Part model, mm, in its own coordinate system. Face numbers are marked on the shaded views. A direction names the side the tool comes from. Round coordinates to 2 decimals unless told otherwise and drop trailing zeros. Loops run counter-clockwise (first coordinate to the right, second up) from the corner with the lowest first, then second, coordinate; pieces in that order, holes last.
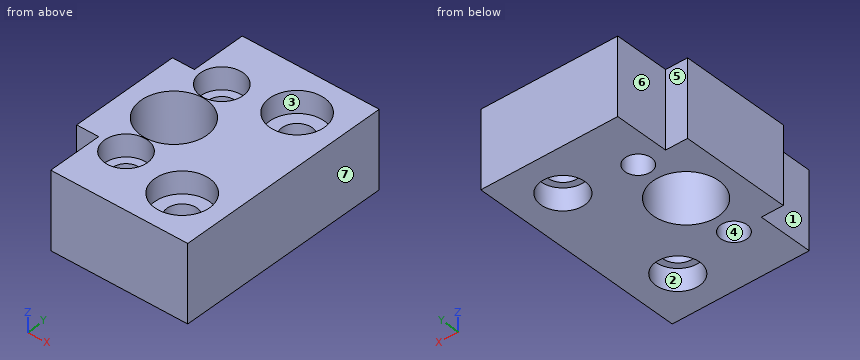
Autodesk Inventor part; units mm, degrees
ref_plane "YZ Plane" through (0, 0, 0) normal (1, 0, 0) x (0, 1, 0)
ref_plane "XZ Plane" through (0, 0, 0) normal (0, 1, 0) x (-1, 0, 0)
ref_plane "XY Plane" through (0, 0, 0) normal (0, 0, 1) x (1, 0, 0)
sketch "Sketch1" plane through (0, 0, 0) normal (0, 0, 1) x (1, 0, 0)
  line L0 (10, -10) -> (-10, -10)
  line L1 (-10, -10) -> (-10, 10)
  line L2 (-10, 10) -> (10, 10)
  line L3 (10, 10) -> (10, -10)
  circle A0 centre (0, 5) radius 1.2
  circle A1 centre (0, -5) radius 1.2
  circle A2 centre (0, 0) radius 3
  dimension "d0" = 10
  dimension "d1" = 10
  dimension "d2" = 10
  dimension "d3" = 10
  dimension "d4" = 5
  dimension "d5" = 5
  dimension "d6" = 2.4
  dimension "d7" = 2.4
  dimension "d8" = 6
extrude "Extrusion1" add sketch "Sketch1" along normal blind 5
sketch "Sketch2" plane through (0, 0, 5) normal (0, 0, 1) x (1, 0, 0)
  line L0 (0, 0) -> (-1.3346, -1.3533)
  circle A0 centre (6, -6) radius 2.5
  circle A1 centre (6, 6) radius 2.5
  line L1 (10, -10) -> (10, 10)
  line L2 (-10, -10) -> (10, -10)
  line L3 (10, 10) -> (-10, 10)
  dimension "d34" = 4
  dimension "d35" = 4
  dimension "d36" = 4
  dimension "d37" = 4
  dimension "d38" = 5
  dimension "d39" = 5
extrude "Extrusion2" cut sketch "Sketch2" against normal blind 1
sketch "Sketch7" plane through (0, 0, 0) normal (0, 0, -1) x (-1, 0, 0)
  circle A0 centre (-6, 6) radius 2.5
  circle A1 centre (-6, 6) radius 1.375
  circle A2 centre (-6, -6) radius 2.5
  circle A3 centre (-6, -6) radius 1.375
  point P0 (0, 0)
  dimension "d40" = 2.75
  dimension "d41" = 2.75
extrude "Extrusion6" cut sketch "Sketch7" against normal blind 5 contours A1 | A3
sketch "Sketch8" plane through (0, 0, 5) normal (0, 0, 1) x (1, 0, 0)
  line L0 (10, 10) -> (-10, 10)
  line L1 (10, 10) -> (2.5, 10)
  line L2 (2.5, 10) -> (2.5, 2.5)
  line L3 (2.5, 2.5) -> (10, 2.5)
  line L4 (10, 2.5) -> (10, 10)
  line L5 (10, -10) -> (10, 10)
  line L6 (10, -10) -> (2.5, -10)
  line L7 (2.5, -10) -> (2.5, -2.5)
  line L8 (2.5, -2.5) -> (10, -2.5)
  line L9 (10, -2.5) -> (10, -10)
  line L10 (10, -2.5) -> (5, -2.5)
  line L11 (5, -2.5) -> (5, 2.5)
  line L12 (5, 2.5) -> (10, 2.5)
  line L13 (10, 2.5) -> (10, -2.5)
  circle A0 centre (6, 6) radius 2.5
  circle A1 centre (6, 6) radius 2.5
  circle A2 centre (6, -6) radius 2.5
  circle A3 centre (6, -6) radius 2.5
  point P0 (0, 0)
  point P1 (2.5, 10)
  dimension "d44" = 7.5
  dimension "d45" = 7.5
  dimension "d46" = 7.5
  dimension "d47" = 7.5
  dimension "d48" = 5
extrude "Extrusion7" add sketch "Sketch8" along normal blind 2
sketch "Sketch9" plane through (0, 0, 0) normal (0, 0, -1) x (-1, 0, 0)
  circle A0 centre (-6, 6) radius 1.375
  circle A1 centre (-6, 6) radius 2
  circle A2 centre (-6, -6) radius 1.375
  circle A3 centre (-6, -6) radius 2
  point P0 (0, 0)
  dimension "d51" = 4
  dimension "d52" = 4
extrude "Extrusion8" cut sketch "Sketch9" against normal blind 2 contours A0 | A1 | A2 | A3
sketch "Sketch10" plane through (0, 0, 0) normal (0, 0, -1) x (-1, 0, 0)
  line L0 (-2.5, 10) -> (10, 10)
  line L1 (10, -10) -> (-2.5, -10)
  line L2 (10, 10) -> (5, 10)
  line L3 (5, 10) -> (5, -10)
  line L4 (5, -10) -> (10, -10)
  line L5 (10, -10) -> (10, 10)
  line L6 (5, 10) -> (2.5, 10)
  line L7 (2.5, 10) -> (2.5, 5)
  line L8 (2.5, 5) -> (5, 5)
  line L9 (5, 5) -> (5, 10)
  line L10 (5, -10) -> (2.5, -10)
  line L11 (2.5, -10) -> (2.5, -5)
  line L12 (2.5, -5) -> (5, -5)
  line L13 (5, -5) -> (5, -10)
  point P0 (0, 0)
  point P1 (2.5, 10)
  dimension "d55" = 5
  dimension "d56" = 2.5
  dimension "d57" = 5
  dimension "d58" = 5
  dimension "d59" = 2.5
extrude "Extrusion9" cut sketch "Sketch10" against normal blind 10
sketch "Sketch12" plane through (6, -6, 4) normal (0, 0, 1) x (1, 0, 0)
  circle A0 centre (0, 0) radius 1.375
  circle A1 centre (0, 0) radius 2.5
  circle A2 centre (0, 12) radius 2
  circle A3 centre (0, 12) radius 1.375
  circle A4 centre (0, 12) radius 2.5
  point P0 (-6, 6)
extrude "Extrusion11" add sketch "Sketch12" along normal blind 1 contours A1 | A2 | A4
sketch "Sketch13" plane through (0, 0, 5) normal (0, 0, 1) x (1, 0, 0)
  point P0 (0, 0)
sketch "Sketch14" plane through (0, 0, 5) normal (0, 0, 1) x (1, 0, 0)
  line L0 (-2.5, -5) -> (-2.5, -10)
  line L1 (-2.5, -10) -> (2.5, -10)
  line L2 (2.5, -10) -> (2.5, -2.5)
  line L3 (2.5, -2.5) -> (5, -2.5)
  line L4 (5, -2.5) -> (5, 2.5)
  line L5 (5, 2.5) -> (2.5, 2.5)
  line L6 (2.5, 2.5) -> (2.5, 10)
  line L7 (2.5, 10) -> (-2.5, 10)
  line L8 (-2.5, 10) -> (-2.5, 5)
  line L9 (-2.5, 5) -> (-5, 5)
  line L10 (-5, 5) -> (-5, -5)
  line L11 (-5, -5) -> (-2.5, -5)
  circle A0 centre (0, 0) radius 3
  circle A1 centre (0, -5) radius 1.2
  circle A2 centre (0, 5) radius 1.2
  circle A3 centre (0, -5) radius 1.95
  circle A4 centre (0, 5) radius 1.95
  dimension "d80" = 3.9
  dimension "d81" = 3.9
extrude "Extrusion12" add sketch "Sketch14" along normal blind 2 contours L11 L10 L9 L8 L7 L6 L5 L4 L3 L2 L1 L0
sketch "Sketch15" plane through (-5, -5, 0) normal (-1, 0, 0) x (0, 0, 1)
  line L0 (0, 10) -> (7, 10)
  line L1 (0, 0) -> (0, 10)
  line L2 (0, 0) -> (7, 0)
  line L3 (7, 10) -> (7, 0)
  point P0 (0, 5)
extrude "Extrusion13" cut sketch "Sketch15" against normal blind 0.5
equation "\"d7\" = d6"
equation "\"d39\" = d38"
equation "\"d45\" = d44"
equation "\"d46\" = d45"
equation "\"d52\" = d51"
equation "\"d81\" = d80"
properties part number "MotorMount"
1) Slice it at D-D, the plane y = -2. Give the cut face in (x, z).
Values:
outline: (-4.5, 0) - (-2.24, 0) - (-2.24, 7) - (-4.5, 7) - close; (2.24, 0) - (10, 0) - (10, 7) - (2.24, 7) - close
2) Drop flat-ended pins along their axis: pin 1 Ø3.5 at (x, y) = (6, 6) entering from -Z; pin 2 Ø3 at (x, y) = (0, -5) entering from +Z; pin 3 Ø5 at (x, y) = (0, 0) entering from -Z; pin 4 Ø1.5 at (y, z) = (6.5, 2.5) entering from -X. Give the stop position or say it passes through.
Values:
pin 1: stops at z = 2
pin 2: stops at z = 5
pin 3: passes through
pin 4: stops at x = -2.5
3) Tool access for the marked faces 1, 2 and 3: list every direction of +Z, -Z, +X, -X, +Y, -Y with a clear straight run to the whole face (end or side of a thin tool).
Values:
face 1: +Z, -Z, -X, -Y
face 2: -Z
face 3: +Z
4) Slice it at C-C, the plane x = 6. Give the cut face in (y, z) (3 decimals), then the cut area to 3 significant figures.
Values:
outline: (-10, 0) - (-8, 0) - (-8, 2) - (-7.375, 2) - (-7.375, 5) - (-8.5, 5) - (-8.5, 7) - (-10, 7) - close; (-4.625, 2) - (-4, 2) - (-4, 0) - (4, 0) - (4, 2) - (4.625, 2) - (4.625, 5) - (3.5, 5) - (3.5, 7) - (-3.5, 7) - (-3.5, 5) - (-4.625, 5) - close; (7.375, 2) - (8, 2) - (8, 0) - (10, 0) - (10, 7) - (8.5, 7) - (8.5, 5) - (7.375, 5) - close
area: 87.5 mm2
5) Mould opens along X. For the marked faces 4, 5, 6 and 7 say: released by +X, released by -X, zero draft, split by the parting line, or undercut.
Values:
face 4: undercut
face 5: zero draft
face 6: released by -X
face 7: released by +X
6) Slice it at A-A, the plane x = 0. Give the cut face in (y, z), then the cut area to 3 significant figures.
Values:
outline: (-10, 0) - (-6.2, 0) - (-6.2, 5) - (-6.95, 5) - (-6.95, 7) - (-10, 7) - close; (-3.8, 0) - (-3, 0) - (-3, 7) - (-3.05, 7) - (-3.05, 5) - (-3.8, 5) - close; (3, 0) - (3.8, 0) - (3.8, 5) - (3.05, 5) - (3.05, 7) - (3, 7) - close; (6.2, 0) - (10, 0) - (10, 7) - (6.95, 7) - (6.95, 5) - (6.2, 5) - close
area: 58.4 mm2
7) Slice it at B-B, the plane z = 4.75. Give the cut face in (x, y) (3 decimals), then the cut area to 3 significant figures.
Values:
outline: (-4.5, -5) - (-2.5, -5) - (-2.5, -10) - (10, -10) - (10, 10) - (-2.5, 10) - (-2.5, 5) - (-4.5, 5) - close; hole circle Ø6 at (0, 0); hole circle Ø2.4 at (0, -5); hole circle Ø2.4 at (0, 5); hole circle Ø2.75 at (6, -6); hole circle Ø2.75 at (6, 6)
area: 221 mm2
8) Wall check: line 1 along Y through (x, z) = (6, 4.2) (3 decimals); line 2 along Y through (x, z) = (6, 0.55); line 3 along Y through (x, z) = (0, 1.5). Give the ranges that are in metal, low to high.
Values:
line 1: y = -10 to -7.375, -4.625 to 4.625, 7.375 to 10
line 2: y = -10 to -8, -4 to 4, 8 to 10
line 3: y = -10 to -6.2, -3.8 to -3, 3 to 3.8, 6.2 to 10
